Autodesk Inventor part; units mm, degrees
ref_plane "YZ Plane" through (0, 0, 0) normal (1, 0, 0) x (0, 1, 0)
ref_plane "XZ Plane" through (0, 0, 0) normal (0, 1, 0) x (-1, 0, 0)
ref_plane "XY Plane" through (0, 0, 0) normal (0, 0, 1) x (1, 0, 0)
sketch "Sketch6" plane through (0, 0, 0) normal (0, 1, 0) x (-1, 0, 0)
  line L0 (0, 0) -> (12, 0)
  line L1 (12, 0) -> (12, -34.549)
  line L2 (12, -34.549) -> (0, -34.549)
  line L3 (0, -34.549) -> (0, 0)
  dimension "d22" = 12
  dimension "d23" = 34.549
extrude "Extrusion6" add sketch "Sketch6" along normal blind 4
sketch "Sketch7" plane through (0, 4, 0) normal (0, 1, 0) x (1, 0, 0)
  line L0 (-12, 0) -> (0, 0)
  line L1 (0, 0) -> (-6, 0)
  line L2 (-6, 0) -> (-6, 10.7)
  line L3 (-6, 10.7) -> (0, 10.7)
  line L4 (0, 10.7) -> (0, 0)
  circle A0 centre (-6, 10.7) radius 2.5
  dimension "d26" = 6
  dimension "d27" = 10.7
  dimension "d28" = 5
extrude "Extrusion7" add sketch "Sketch7" along normal blind 6 contours A0 L3 L2 | L2 L3 A0
properties part number "filler"
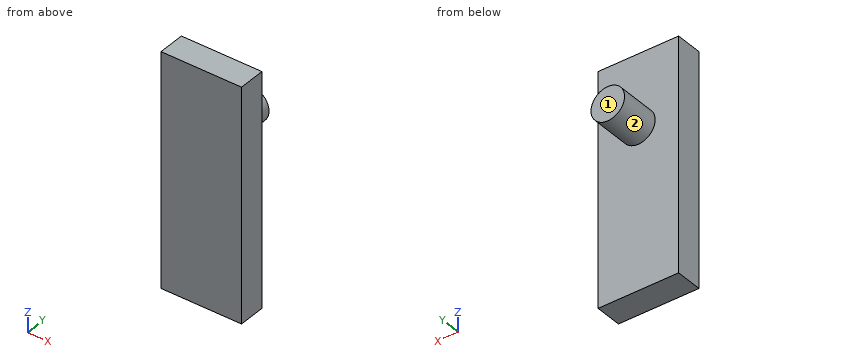
Can you work these out from the model? Positions are in its coordinate system, mm. Face numbers are marked on the shaded views. A direction names the side the tool comes from. Coordinates: 2 decimals unless noted, no trailing zeros. Order: outer loops, then holes, each group sorted by start corner. A loop starts at its lowest first (then second) coordinate and runs counter-clockwise, first axis right, second up.
1. If we section it at A-A (z = -10.7): Please give me the cut outline in (x, y), then the cut area to 3 significant figures.
2. I'm going to push flat-ended pins straight in: pin 1 (5 mm diameter, centred on y = 7.5, z = -21.5, fed in from +X); pin 2 (3 mm diameter, centred on x = -6.5, y = 7.5, fed in from -Z); pin 3 (6 mm diameter, centred on x = -4.5, z = -25.5, fed in from +Y). Where does each tip first touch, or does it pass through?
3. I need wall thicknesses on line 1 (Y direction, x = -6.25, z = -16); line 2 (Z direction, x = -4, y = 4.75); line 3 (X direction, y = 6.5, z = -9). Which ranges of each line are inside material? Lowest first, please.
4. If we section it at C-C (y = 7): Please give me the cut outline in (x, z), then the cut area to 3 significant figures.
5. If we section it at B-B (x = -6): Please give me the cut outline in (y, z), then the cut area to 3 significant figures.
6. For the marked faces 1 and 2, which set-ups out of +Z, -Z, +X, -X, +Y, -Y let a thin tool reach every point of the face, with its end or its side?
7. If we section it at D-D (z = -7): Please give me the cut outline in (x, y).
Entries:
1. outline: (-12, 0) - (0, 0) - (0, 4) - (-3.5, 4) - (-3.5, 10) - (-8.5, 10) - (-8.5, 4) - (-12, 4) - close
1. area: 78.0 mm2
2. pin 1: passes through
2. pin 2: stops at z = -13.2
2. pin 3: stops at y = 4
3. line 1: y = 0 to 4
3. line 2: z = -12.2 to -9.2
3. line 3: x = -7.83 to -4.17
4. outline: circle Ø5 at (-6, -10.7)
4. area: 19.6 mm2
5. outline: (0, -34.55) - (4, -34.55) - (4, -13.2) - (10, -13.2) - (10, -8.2) - (4, -8.2) - (4, 0) - (0, 0) - close
5. area: 168 mm2
6. face 1: +Z, -Z, +X, -X, +Y
6. face 2: +Y
7. outline: (-12, 0) - (0, 0) - (0, 4) - (-12, 4) - close
